Input: dimensioned drawing with shaded views. Units: mm. Origin: part minimum x, y, z. Give positions to 0.01 mm unless a question says otherwise; leave off trailing zeros. Write each loop counter-clockwise with the first axis right and the second up, starting at its lowest first coordinate (ties: lowest second). Pieces come first, ordered by that corner, then holes.
Q1. Line query: line 1 (Z direction, x = 7.5, y = 0.1); line 2 (X direction, y = 1, z = 20); line 3 (Z direction, x = 1.5, y = 1) (1 decimal). Output: solid intervals per line, ascending.
Q2. Section C-C (y = 0.75). State how many separate pieces and enclosed holes the cut face has, plus the area to 3 significant figures.
Q3. Pin query (flat end, axial travel): pin 1 Ø6 at (x, z) = (7, 22.5) entering from -Y. Return the tip coordinate at first contact, or that it passes through.
Q4. Section B-B (x = 6.25). Return the cut outline in (y, z).
Q5. Section D-D (z = 14). Return the cut outline in (x, y), plus the area to 3 significant figures.
Q6. Section A-A (z = 32.5). Return the cut outline in (x, y).
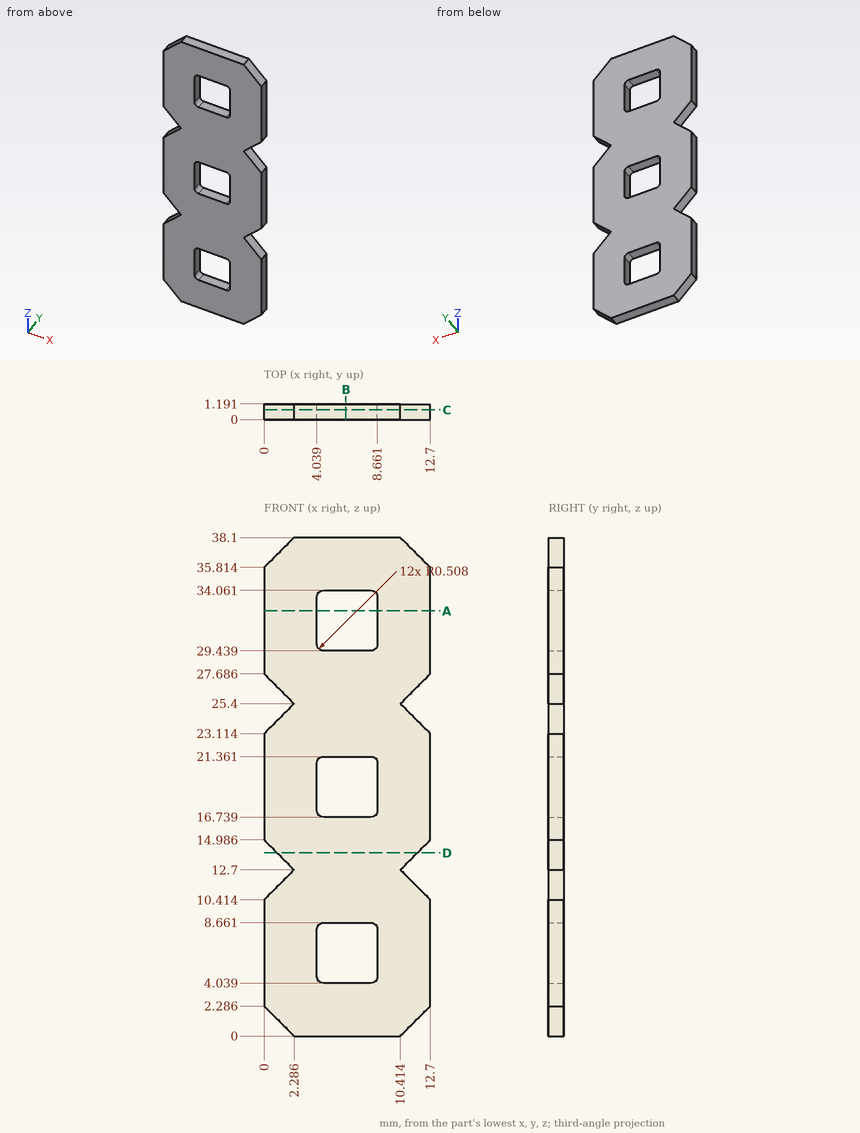
Computed:
1. line 1: z = 0 to 4.04, 8.66 to 16.74, 21.36 to 29.44, 34.06 to 38.1
1. line 2: x = 0 to 4.04, 8.66 to 12.7
1. line 3: z = 0.8 to 11.9, 13.5 to 24.6, 26.2 to 37.3
2. separate pieces: 1
2. enclosed holes: 3
2. area: 389 mm2
3. pin 1: stops at y = 0
4. outline: (0, 0) - (1.19, 0) - (1.19, 4.04) - (0, 4.04) - close; (0, 8.66) - (1.19, 8.66) - (1.19, 16.74) - (0, 16.74) - close; (0, 21.36) - (1.19, 21.36) - (1.19, 29.44) - (0, 29.44) - close; (0, 34.06) - (1.19, 34.06) - (1.19, 38.1) - (0, 38.1) - close
5. outline: (0.99, 0) - (11.71, 0) - (11.71, 1.19) - (0.99, 1.19) - close
5. area: 12.8 mm2
6. outline: (0, 0) - (4.04, 0) - (4.04, 1.19) - (0, 1.19) - close; (8.66, 0) - (12.7, 0) - (12.7, 1.19) - (8.66, 1.19) - close
